Drawing for the job (mm, zero at the part's lowest x, y, z). Round coordinates to 2 decimals unless told otherwise and drop trailing zeros. Write each loop counter-clockwise with the first axis right and the second up, starting at its lowest first coordinate (ties: lowest second). Pieces come first, ordered by that corner, then holes.
Item 1: Band-saw the part on C-C, the plane z = 5. Write the cut outline in (x, y) (1 decimal).
Item 2: Wall check: probe 1 along Z at (x, y) = (96.5, 32.5); probe 2 along Y at (x, z) = (17, 5) (1 decimal); probe 3 along X at (y, z) = (37, 19) (1 decimal). Give the ranges that are in metal, low to high.
Item 3: Drop flat-ended pins along their axis: pin 1 Ø1.9 at (x, z) = (49, 1.5) entering from +Y; pin 2 Ø7 at (y, z) = (22.5, 1.5) entering from -X; pin 3 Ø3 at (y, z) = (44.5, 2.5) entering from +X. Give the stop position or say it passes through.
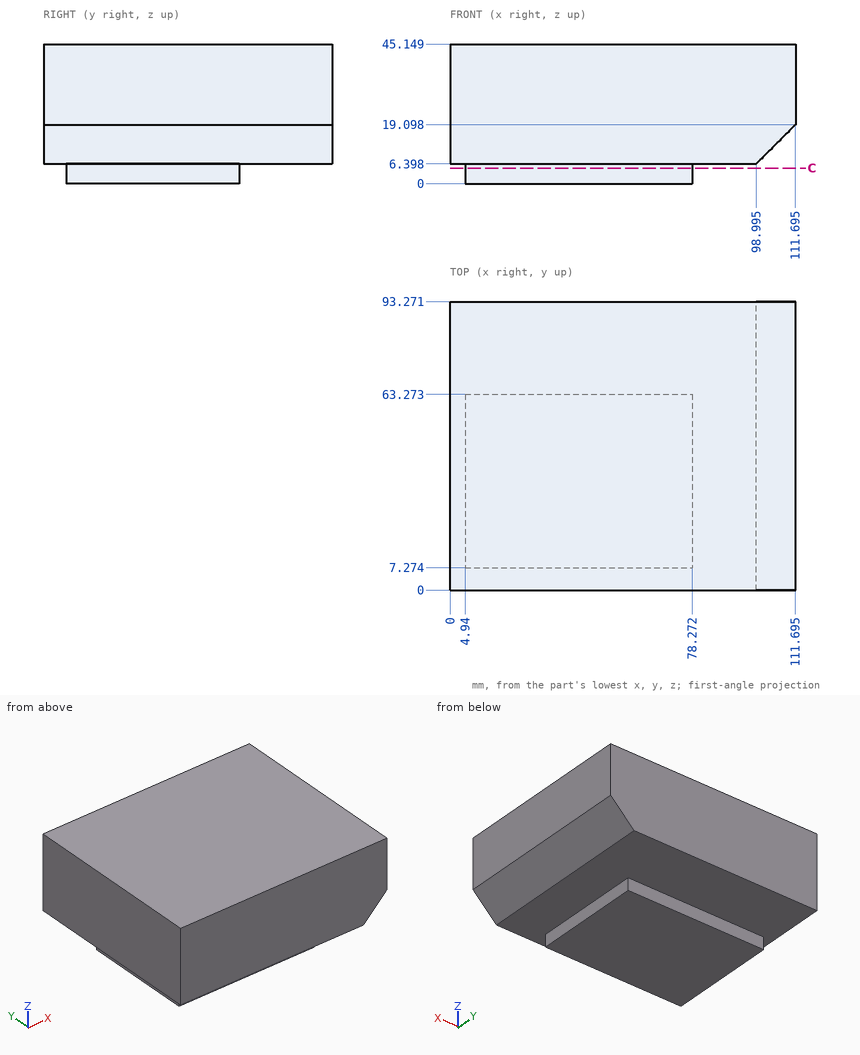
Results:
1. outline: (4.9, 7.3) - (78.3, 7.3) - (78.3, 63.3) - (4.9, 63.3) - close
2. probe 1: z = 6.4 to 45.15
2. probe 2: y = 7.3 to 63.3
2. probe 3: x = 0 to 111.6
3. pin 1: stops at y = 63.27
3. pin 2: stops at x = 4.94
3. pin 3: stops at x = 78.27
